The model under review builds one solid part; all positions refer to its coordinate system, in mm. A direction names the side the tool comes from. Give positions to 0.01 mm unless a question says otherwise; leave off trailing zeros. Order: outer loops, then holes, each group sorted by start corner. A loop starts at its lowest first (then second) coordinate and runs counter-clockwise, first axis right, second up.
```python
from build123d import *

# Parameters (mm, degrees)
BOSS_EXTRUDE1_DEPTH = 590
CUT_EXTRUDE3_REACH  = 5
SKETCH2_R           = 2.55
CUT_EXTRUDE5_REACH  = 5
SKETCH5_W           = 55
SKETCH5_H           = 20
CUT_EXTRUDE6_REACH  = 12
SKETCH6_R           = 2.55


with BuildPart() as part:
    # Sketch1 → Boss-Extrude1 (new body)
    with BuildSketch(Plane.XY):
        Polygon((0, 0), (0, 40), (10, 40), (10, 37), (3, 37), (3, 0), align=None)
    extrude(amount=BOSS_EXTRUDE1_DEPTH)

    # Sketch2 → Cut-Extrude3 (cut, up to next)
    with BuildSketch(Plane(origin=(3, 0, 0), x_dir=(0, 0, -1), z_dir=(1, 0, 0)), mode=Mode.PRIVATE) as cut_extrude3_sk1:
        with Locations((-525, 10)):
            Circle(SKETCH2_R)
    cut_extrude3_tool1 = extrude(cut_extrude3_sk1.sketch, amount=-CUT_EXTRUDE3_REACH, mode=Mode.PRIVATE) & part.part
    add(cut_extrude3_tool1.solids().sort_by_distance((3, 10, 525))[0], mode=Mode.SUBTRACT)
    # Sketch2 → Cut-Extrude3 (cut, up to next)
    with BuildSketch(Plane(origin=(3, 0, 0), x_dir=(0, 0, -1), z_dir=(1, 0, 0)), mode=Mode.PRIVATE) as cut_extrude3_sk2:
        with Locations((-295, 10)):
            Circle(SKETCH2_R)
    cut_extrude3_tool2 = extrude(cut_extrude3_sk2.sketch, amount=-CUT_EXTRUDE3_REACH, mode=Mode.PRIVATE) & part.part
    add(cut_extrude3_tool2.solids().sort_by_distance((3, 10, 295))[0], mode=Mode.SUBTRACT)
    # Sketch2 → Cut-Extrude3 (cut, up to next)
    with BuildSketch(Plane(origin=(3, 0, 0), x_dir=(0, 0, -1), z_dir=(1, 0, 0)), mode=Mode.PRIVATE) as cut_extrude3_sk3:
        with Locations((-415, 10)):
            Circle(SKETCH2_R)
    cut_extrude3_tool3 = extrude(cut_extrude3_sk3.sketch, amount=-CUT_EXTRUDE3_REACH, mode=Mode.PRIVATE) & part.part
    add(cut_extrude3_tool3.solids().sort_by_distance((3, 10, 415))[0], mode=Mode.SUBTRACT)
    # Sketch2 → Cut-Extrude3 (cut, up to next)
    with BuildSketch(Plane(origin=(3, 0, 0), x_dir=(0, 0, -1), z_dir=(1, 0, 0)), mode=Mode.PRIVATE) as cut_extrude3_sk4:
        with Locations((-175, 10)):
            Circle(SKETCH2_R)
    cut_extrude3_tool4 = extrude(cut_extrude3_sk4.sketch, amount=-CUT_EXTRUDE3_REACH, mode=Mode.PRIVATE) & part.part
    add(cut_extrude3_tool4.solids().sort_by_distance((3, 10, 175))[0], mode=Mode.SUBTRACT)
    # Sketch2 → Cut-Extrude3 (cut, up to next)
    with BuildSketch(Plane(origin=(3, 0, 0), x_dir=(0, 0, -1), z_dir=(1, 0, 0)), mode=Mode.PRIVATE) as cut_extrude3_sk5:
        with Locations((-65, 10)):
            Circle(SKETCH2_R)
    cut_extrude3_tool5 = extrude(cut_extrude3_sk5.sketch, amount=-CUT_EXTRUDE3_REACH, mode=Mode.PRIVATE) & part.part
    add(cut_extrude3_tool5.solids().sort_by_distance((3, 10, 65))[0], mode=Mode.SUBTRACT)

    # Sketch5 → Cut-Extrude5 (cut, up to next)
    with BuildSketch(Plane(origin=(3, 0, 0), x_dir=(0, 0, -1), z_dir=(1, 0, 0)), mode=Mode.PRIVATE) as cut_extrude5_sk1:
        with Locations((-562.5, 10)):
            Rectangle(SKETCH5_W, SKETCH5_H)
    cut_extrude5_tool1 = extrude(cut_extrude5_sk1.sketch, amount=-CUT_EXTRUDE5_REACH, mode=Mode.PRIVATE) & part.part
    add(cut_extrude5_tool1.solids().sort_by_distance((3, 10, 562.5))[0], mode=Mode.SUBTRACT)
    # Sketch5 → Cut-Extrude5 (cut, up to next)
    with BuildSketch(Plane(origin=(3, 0, 0), x_dir=(0, 0, -1), z_dir=(1, 0, 0)), mode=Mode.PRIVATE) as cut_extrude5_sk2:
        with Locations((-27.5, 10)):
            Rectangle(SKETCH5_W, SKETCH5_H)
    cut_extrude5_tool2 = extrude(cut_extrude5_sk2.sketch, amount=-CUT_EXTRUDE5_REACH, mode=Mode.PRIVATE) & part.part
    add(cut_extrude5_tool2.solids().sort_by_distance((3, 10, 27.5))[0], mode=Mode.SUBTRACT)

    # Sketch6 → Cut-Extrude6 (cut, up to next)
    with BuildSketch(Plane.ZY, mode=Mode.PRIVATE) as cut_extrude6_sk1:
        with Locations((10, 30)):
            Circle(SKETCH6_R)
    cut_extrude6_tool1 = extrude(cut_extrude6_sk1.sketch, amount=-CUT_EXTRUDE6_REACH, mode=Mode.PRIVATE) & part.part
    add(cut_extrude6_tool1.solids().sort_by_distance((0, 30, 10))[0], mode=Mode.SUBTRACT)
    # Sketch6 → Cut-Extrude6 (cut, up to next)
    with BuildSketch(Plane.ZY, mode=Mode.PRIVATE) as cut_extrude6_sk2:
        with Locations((580, 30)):
            Circle(SKETCH6_R)
    cut_extrude6_tool2 = extrude(cut_extrude6_sk2.sketch, amount=-CUT_EXTRUDE6_REACH, mode=Mode.PRIVATE) & part.part
    add(cut_extrude6_tool2.solids().sort_by_distance((0, 30, 580))[0], mode=Mode.SUBTRACT)
    # Sketch6 → Cut-Extrude6 (cut, up to next)
    with BuildSketch(Plane.ZY, mode=Mode.PRIVATE) as cut_extrude6_sk3:
        with BuildLine():
            Line((30, 32.55), (50, 32.55))
            ThreePointArc((50, 32.55), (52.55, 30), (50, 27.45))
            Line((50, 27.45), (30, 27.45))
            ThreePointArc((30, 27.45), (27.45, 30), (30, 32.55))
        make_face()
    cut_extrude6_tool3 = extrude(cut_extrude6_sk3.sketch, amount=-CUT_EXTRUDE6_REACH, mode=Mode.PRIVATE) & part.part
    add(cut_extrude6_tool3.solids().sort_by_distance((0, 30, 40))[0], mode=Mode.SUBTRACT)
    # Sketch6 → Cut-Extrude6 (cut, up to next)
    with BuildSketch(Plane.ZY, mode=Mode.PRIVATE) as cut_extrude6_sk4:
        with BuildLine():
            Line((560, 32.55), (540, 32.55))
            ThreePointArc((540, 32.55), (537.45, 30), (540, 27.45))
            Line((540, 27.45), (560, 27.45))
            ThreePointArc((560, 27.45), (562.55, 30), (560, 32.55))
        make_face()
    cut_extrude6_tool4 = extrude(cut_extrude6_sk4.sketch, amount=-CUT_EXTRUDE6_REACH, mode=Mode.PRIVATE) & part.part
    add(cut_extrude6_tool4.solids().sort_by_distance((0, 30, 550))[0], mode=Mode.SUBTRACT)


solid = part.part
```
1. For faces 1 (the flat face through (3, 19, 291)), 2 (the flat face through (5, 40, 291)), list the 3-axis set-ups (+Z, -Z, +X, -X, +Y, -Y) from which the entire face can be reached by the end or side of a thin tool; tool diameter is ignored.
2. Take a section at B-B (x = 6). Write out the cut boundary in (y, z).
3. Take a section at A-A (z = 425.5). Write out the cut boundary in (x, y).
4. Insertion check: pin 1 (1.5 mm diameter, centred on x = 1.5, z = 558.5, fed in from -Y); pin 2 (18.5 mm diameter, centred on y = 16, z = 421, fed in from +X); pin 3 (1.5 mm diameter, centred on x = 2.5, y = 18, fed in from +Z). Each pin has a flat end and moves straight along its axis. Give the tip position at first contact, or say it passes through.
5. To check wall thickness, follow line 1 (Y direction, x = 0.6, z = 10); line 2 (Y direction, x = 0.95, z = 175); line 3 (X direction, y = 12, z = 230). State the ranges of each line that lie inside material, in increasing order.
Answer:
1. face 1: +Z, -Z, +X, -Y
1. face 2: +Z, -Z, +X, -X, +Y
2. outline: (37, 0) - (40, 0) - (40, 590) - (37, 590) - close
3. outline: (0, 0) - (3, 0) - (3, 37) - (10, 37) - (10, 40) - (0, 40) - close
4. pin 1: stops at y = 20
4. pin 2: stops at x = 3
4. pin 3: stops at z = 535
5. line 1: y = 20 to 27.45, 32.55 to 40
5. line 2: y = 0 to 7.45, 12.55 to 40
5. line 3: x = 0 to 3
